Check sheet for the drawn part. Datum: minimum x, y, z corner. Units: mm. Give positions to 0.01 mm unless a question says otherwise; leave off trailing zeros. Write each loop counter-clockwise with the first axis right and the second up, starting at its lowest first coordinate (ties: lowest second). Pieces come first, ordered by that corner, then holes. Notation, with made-up numbers: (10, -38.5) - (56, -38.5) arc R17 cw to (56, -11.5) - close; hole circle Ø10 at (81, 22.25). An arc over 180 degrees is marked (long way). Answer as a JSON object with one key per item and string values. Group by question number.
Item 1: Go/stop test with a flat-tipped pin: pin 1 (3.5 mm diameter, centred on x = 31.5, y = 4.5, fed in from +Z). Record where the tip stops, or that it passes through.
Item 2: Scan lines: line 1 along Y through (x, z) = (13.5, 1.85); line 2 along X through (y, z) = (41.5, 0.3); line 3 along X through (y, z) = (50, 2.3). Record each from-to range of solid material in increasing order. Write a range as [from, to].
Item 3: Sectioned sample at D-D, the plane z = 1.5. Count the separate pieces of the cut face and the enclosed holes in it, and give its area (3 significant figures).
Item 4: Sectioned sample at A-A, the plane y = 49.5. Record the boundary of the cut face in (x, z), and give its area (3 significant figures).
Item 5: Sectioned sample at B-B, the plane x = 31.5. Record the boundary of the cut face in (y, z), and give its area (3 significant figures).
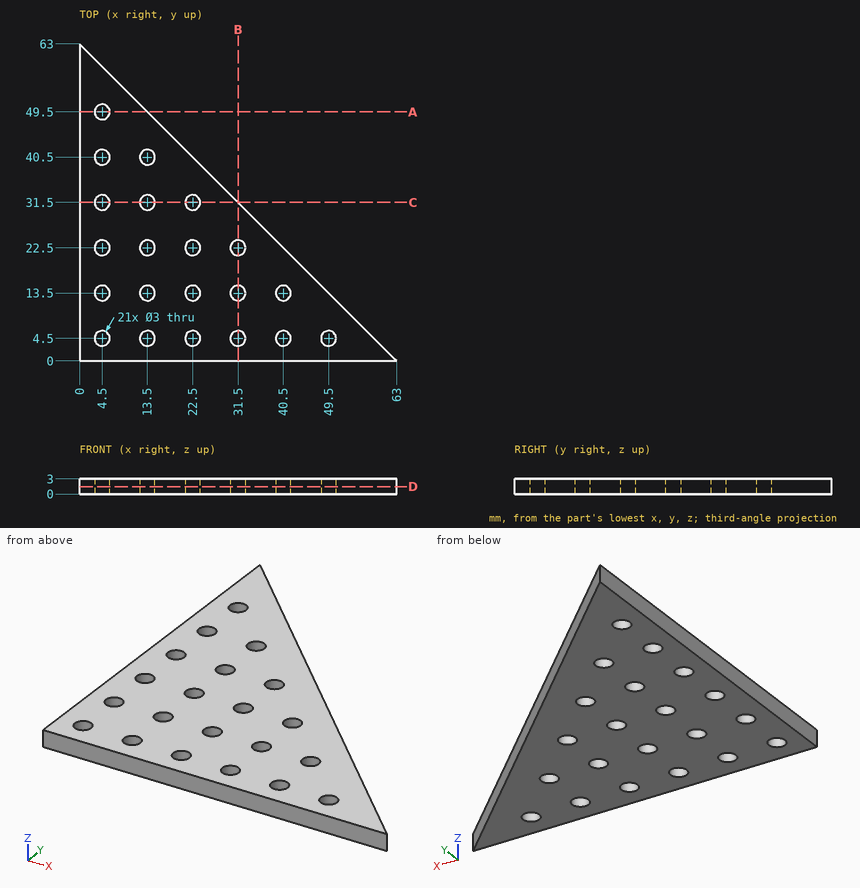
Geometry check:
{
 "1": {"pin 1": "z = 3"},
 "2": {"line 1": "[0, 3], [6, 12], [15, 21], [24, 30], [33, 39], [42, 49.5]", "line 2": "[0, 3.38], [5.62, 12.38], [14.62, 21.5]", "line 3": "[0, 3.09], [5.91, 13]"},
 "3": {"separate pieces": "1", "enclosed holes": "21", "area": "1,840 mm^2"},
 "4": {"outline": "(0, 0) - (3, 0) - (3, 3) - (0, 3) - close; (6, 0) - (13.5, 0) - (13.5, 3) - (6, 3) - close", "area": "31.5 mm^2"},
 "5": {"outline": "(0, 0) - (3, 0) - (3, 3) - (0, 3) - close; (6, 0) - (12, 0) - (12, 3) - (6, 3) - close; (15, 0) - (21, 0) - (21, 3) - (15, 3) - close; (24, 0) - (31.5, 0) - (31.5, 3) - (24, 3) - close", "area": "67.5 mm^2"}
}
